Could you check a few things on this model? Use its own coordinates, in mm. Face numbers are marked on the shaded views. A direction names the side the tool comes from. Give positions to 0.01 mm unless a question says otherwise; leave off trailing zeros. Write each loop counter-clockwise with the first axis right and the second up, starting at its lowest first coordinate (ties: lowest second). Pieces come first, ordered by that corner, then holes. Notation, with made-up numbers: M -16,13.5 L 32,13.5 A32 ccw 32,41.5 Z; hole C -23,-1 d4. An arc over 180 degrees is marked long. Use one line per item in the form item = value.
from build123d import *

# Parameters (mm, degrees)
SKETCH1_W                                       = 152.4
SKETCH1_H                                       = 31.75
BOSS_EXTRUDE1_DEPTH                             = 4.7625
CSK_FOR_M3_FLAT_HEAD_MACHINE_SCREW1_D           = 3.2
CSK_FOR_M3_FLAT_HEAD_MACHINE_SCREW1_CSINK_D     = 6.3
CSK_FOR_M3_FLAT_HEAD_MACHINE_SCREW1_CSINK_ANGLE = 90
F_12_0MM_DOWEL_HOLE1_D                          = 12
CBORE_FOR_M3_SHCS1_D                            = 3.4
CBORE_FOR_M3_SHCS1_CBORE_D                      = 4.5
CBORE_FOR_M3_SHCS1_CBORE_DEPTH                  = 2
CUT_EXTRUDE1_DEPTH                              = 79.416715374


with BuildPart() as part:
    # Sketch1 → Boss-Extrude1 (new, symmetric)
    with BuildSketch(Plane(origin=(0, 0, 0), x_dir=(1, 0, 0), z_dir=(0, 1, 0))):
        Rectangle(SKETCH1_W, SKETCH1_H)
    extrude(amount=BOSS_EXTRUDE1_DEPTH, both=True)

    # CSK for M3 Flat Head Machine Screw1 (through all)
    with Locations(Plane(origin=(0, 4.7625, 0), x_dir=(1, 0, 0), z_dir=(0, 1, 0))):
        with Locations((-71.4375, -9.525), (71.4375, -9.525), (71.4375, 9.525), (-71.4375, 9.525)):
            CounterSinkHole(CSK_FOR_M3_FLAT_HEAD_MACHINE_SCREW1_D / 2, CSK_FOR_M3_FLAT_HEAD_MACHINE_SCREW1_CSINK_D / 2, counter_sink_angle=CSK_FOR_M3_FLAT_HEAD_MACHINE_SCREW1_CSINK_ANGLE)

    # Ø12.0mm Dowel Hole1 (through all)
    with Locations(Plane(origin=(0, -4.7625, 0), x_dir=(-1, 0, 0), z_dir=(0, -1, 0))):
        with Locations((0, 0)):
            Hole(F_12_0MM_DOWEL_HOLE1_D / 2)

    # CBORE for M3 SHCS1 (through all)
    with Locations(Plane(origin=(0, -4.7625, 0), x_dir=(-1, 0, 0), z_dir=(0, -1, 0))):
        with Locations((4.7625, -8.248891971), (9.525, 0), (4.7625, 8.248891971), (-4.7625, 8.248891971), (-9.525, 0), (-4.7625, -8.248891971)):
            CounterBoreHole(CBORE_FOR_M3_SHCS1_D / 2, CBORE_FOR_M3_SHCS1_CBORE_D / 2, CBORE_FOR_M3_SHCS1_CBORE_DEPTH)

    # Sketch15 → Cut-Extrude1 (cut, through all)
    with BuildSketch(Plane(origin=(0, 4.7625, 0), x_dir=(1, 0, 0), z_dir=(0, 1, 0))):
        with BuildLine():
            Line((-57.15, 9.525), (-25.4, 9.525))
            ThreePointArc((-25.4, 9.525), (-15.875, 0), (-25.4, -9.525))
            Line((-25.4, -9.525), (-57.15, -9.525))
            ThreePointArc((-57.15, -9.525), (-66.675, 0), (-57.15, 9.525))
        make_face()
        with BuildLine():
            Line((25.4, 9.525), (57.15, 9.525))
            ThreePointArc((57.15, 9.525), (66.675, 0), (57.15, -9.525))
            Line((57.15, -9.525), (25.4, -9.525))
            ThreePointArc((25.4, -9.525), (15.875, 0), (25.4, 9.525))
        make_face()
    extrude(amount=-CUT_EXTRUDE1_DEPTH, mode=Mode.SUBTRACT)


solid = part.part
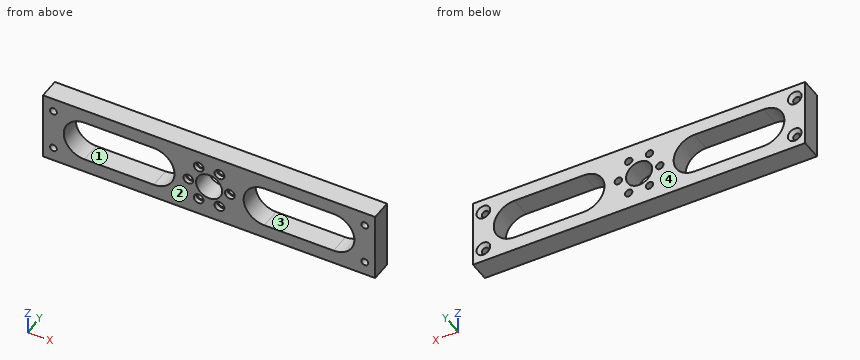
1) Thinking about a two-plate mould opening in X: for the marked faces 1 and 2, which applies, released by +X, released by -X, zero draft, split by the parting line, or undercut?
Checked values:
face_1 = undercut
face_2 = zero draft
2) For the marked faces 3 and 4, which set-ups out of +Z, -Z, +X, -X, +Y, -Y let a thin tool reach every point of the face, with its end or its side?
Checked values:
face_3 = +Y, -Y
face_4 = +Z, -Z, +X, -X, +Y
3) I want a section at D-D, the plane x = -21. Please give me the cut outline in (y, z) (1 decimal), plus the area to 3 significant figures.
Checked values:
outline = M -4.8,-15.9 L 4.8,-15.9 L 4.8,-8.4 L -4.8,-8.4 Z; M -4.8,8.4 L 4.8,8.4 L 4.8,15.9 L -4.8,15.9 Z
area = 141 mm2
4) I want a section at A-A, the plane z = 0. Count the separate pieces of the cut face and the enclosed holes in it, plus the area to 3 significant figures.
Checked values:
separate_pieces = 6
enclosed_holes = 0
area = 300 mm2
5) For pin 1 Ø1.3 at (x, z) = (5, 8.5) entering from -Y; pin 2 Ø4 at (x, z) = (-4.76, 8.25) entering from -Y, each with a flat end and sliding along its axis, tell me the tip position at first contact or that it passes through.
Checked values:
pin_1 = through
pin_2 = -2.76
6) I want a section at B-B, the plane x = 0. Please give me the cut outline in (y, z) (1 decimal).
Checked values:
outline = M -4.8,-15.9 L 4.8,-15.9 L 4.8,-6 L -4.8,-6 Z; M -4.8,6 L 4.8,6 L 4.8,15.9 L -4.8,15.9 Z
7) If I drill on L1, parallel to Z at x = 54, y = 3.5 (3 decimals); L2, parallel to X at y = 2, z = -4; L3, parallel to X at y = -4.25, z = -7.5, over which ranges is the centre line in solid material (lowest first)?
Checked values:
L1 = -15.875 to -9.525, 9.525 to 15.875
L2 = -76.2 to -65.79, -16.76 to -4.47, 4.47 to 16.76, 65.79 to 76.2
L3 = -76.2 to -63.02, -19.53 to -6.88, -2.64 to 2.64, 6.88 to 19.53, 63.02 to 76.2
